Check sheet for the modelled part. Datum: model origin and axes. Units: mm. Face numbers are marked on the shaded views. Give positions to 0.01 mm unless a question says otherwise; leave off trailing zeros. Order: outer loops, then holes, each group sorted by start corner. A loop starts at its lowest first (then second) coordinate and runs counter-clockwise, first axis right, second up. Notation, with made-up numbers: (-29.75, 29) -> (-14.75, 29) arc R27 ccw to (-14.75, 55) -> close; hole circle Ø3 at (-16.75, 23.25). An arc over 180 degrees is marked (long way). One line per question, with ' | ' between items.
```python
from build123d import *

# Parameters (mm, degrees)
BASE_FLANGE1_DEPTH = 304.8
CUT_EXTRUDE3_DEPTH = 350.224373693
SKETCH9_R          = 2.5796875
CUT_EXTRUDE4_DEPTH = 350.224373693


# Sheet-metal steps are written as plain solids
with BuildPart() as part:
    # Sketch1 → Base-Flange1 (new body)
    with BuildSketch(Plane.XY):
        with BuildLine():
            Line((0, 106.68), (0, 4.572))
            ThreePointArc((0, 4.572), (1.339107796, 1.339107796), (4.572, 0))
            Line((4.572, 0), (128.3716, 0))
            ThreePointArc((128.3716, 0), (131.604492204, 1.339107796), (132.9436, 4.572))
            Line((132.9436, 4.572), (132.9436, 106.68))
            Line((132.9436, 106.68), (130.6576, 106.68))
            Line((130.6576, 106.68), (130.6576, 4.572))
            ThreePointArc((130.6576, 4.572), (129.988046102, 2.955553898), (128.3716, 2.286))
            Line((128.3716, 2.286), (4.572, 2.286))
            ThreePointArc((4.572, 2.286), (2.955553898, 2.955553898), (2.286, 4.572))
            Line((2.286, 4.572), (2.286, 106.68))
            Line((2.286, 106.68), (0, 106.68))
        make_face()
    extrude(amount=BASE_FLANGE1_DEPTH)

    # Sketch6 → Cut-Extrude3 (cut, through all)
    with BuildSketch(Plane(origin=(132.9436, 0, 0), x_dir=(0, 0, -1), z_dir=(1, 0, 0))):
        Polygon((0, 4.572), (0, 106.68), (-165.1, 106.68), (-165.1, 30.48), align=None)
    extrude(amount=-CUT_EXTRUDE3_DEPTH, mode=Mode.SUBTRACT)

    # Sketch9 → Cut-Extrude4 (cut, through all)
    with BuildSketch(Plane.ZY):
        with Locations(Location((177.8, 81.28, 0), (0, 0, 270))):
            Circle(SKETCH9_R)
        with Locations(Location((292.1, 81.28, 0), (0, 0, 270))):
            Circle(SKETCH9_R)
    extrude(amount=-CUT_EXTRUDE4_DEPTH, mode=Mode.SUBTRACT)


solid = part.part
```
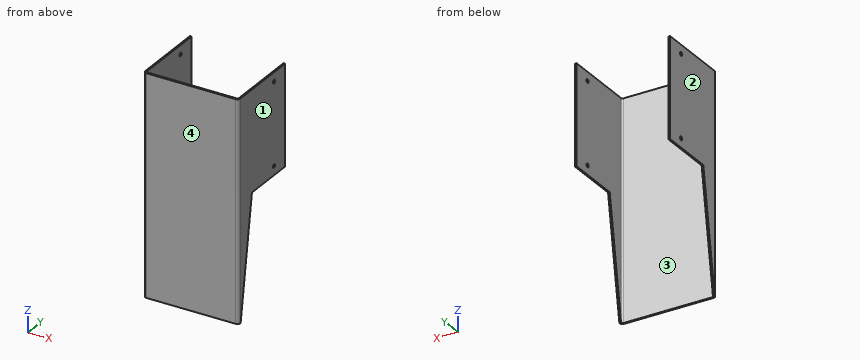
Q1. Thickness scan on line 1 (Z direction, x = 132, y = 81); line 2 (X direction, y = 11, z = 151); line 3 (Y direction, x = 97.5, z = 135). Record the ranges inside material, lowest first.
Result sheet:
line 1: z = 165.1 to 175.24, 180.36 to 289.54, 294.66 to 304.8 | line 2: x = 0 to 2.29, 130.66 to 132.94 | line 3: y = 0 to 2.29
Q2. Section check B-B (z = 260). Enter the section's corners in (x, y).
Result sheet:
outline: (0, 4.57) arc R4.57 ccw to (4.57, 0) -> (128.37, 0) arc R4.57 ccw to (132.94, 4.57) -> (132.94, 106.68) -> (130.66, 106.68) -> (130.66, 4.57) arc R2.29 cw to (128.37, 2.29) -> (4.57, 2.29) arc R2.29 cw to (2.29, 4.57) -> (2.29, 106.68) -> (0, 106.68) -> close
Q3. Section check A-A (y = 62.5). Enter the section's corners in (x, z), and give its area (3 significant figures).
Result sheet:
outline: (0, 165.1) -> (2.29, 165.1) -> (2.29, 304.8) -> (0, 304.8) -> close; (130.66, 165.1) -> (132.94, 165.1) -> (132.94, 304.8) -> (130.66, 304.8) -> close | area: 639 mm2
Q4. Section check C-C (y = 15). Enter the section's corners in (x, z).
Result sheet:
outline: (0, 66.45) -> (2.29, 66.45) -> (2.29, 304.8) -> (0, 304.8) -> close; (130.66, 66.45) -> (132.94, 66.45) -> (132.94, 304.8) -> (130.66, 304.8) -> close
Q5. Depth check by flat-ended pin: pin 1 Ø2.5 at (x, y) = (132, 65.5) entering from -Z; pin 2 Ø2 at (x, z) = (38.5, 61.5) entering from +Y. Enter the tip coordinate at first touch or a pass-through.
Result sheet:
pin 1: stops at z = 165.1 | pin 2: stops at y = 2.29
Q6. Section check D-D (x = 100.5). Enter the section's corners in (y, z).
Result sheet:
outline: (0, 0) -> (2.29, 0) -> (2.29, 304.8) -> (0, 304.8) -> close
Q7. Mould release check, pull along X, two halves, no side actions. Record for the marked faces 1, 2, 3 and 4: pulls with the +X half, pulls with the -X half, needs draft (parallel to the pull), parting line crosses it, or undercut.
Result sheet:
face 1: pulls with the +X half | face 2: pulls with the -X half | face 3: undercut | face 4: needs draft
